```python
from build123d import *

# Parameters (mm, degrees)
SKETCH1_W                = 36
SKETCH1_H                = 120
BOSS_EXTRUDE1_DEPTH      = 1
F_4_0_4_DIAMETER_HOLE2_D = 4
F_4_0_4_DIAMETER_HOLE3_D = 4
F_4_0_4_DIAMETER_HOLE1_D = 4
BOSS_EXTRUDE2_DEPTH      = 1
FILLET1_R                = 4


with BuildPart() as part:
    # Sketch1 → Boss-Extrude1 (new body)
    with BuildSketch(Plane(origin=(0, 0, 0), x_dir=(0, 0, -1), z_dir=(1, 0, 0))):
        with Locations((0, -60)):
            Rectangle(SKETCH1_W, SKETCH1_H)
    extrude(amount=BOSS_EXTRUDE1_DEPTH)

    # Ø4.0 (4) Diameter Hole2 (through all)
    with Locations(Plane.ZY):
        with Locations((-10, -8), (10, -8)):
            Hole(F_4_0_4_DIAMETER_HOLE2_D / 2)

    # Ø4.0 (4) Diameter Hole3 (through all)
    with Locations(Plane.ZY):
        with Locations((-13, -17), (13, -17)):
            Hole(F_4_0_4_DIAMETER_HOLE3_D / 2)

    # Ø4.0 (4) Diameter Hole1 (through all)
    with Locations(Plane(origin=(1, 0, 0), x_dir=(0, 0, -1), z_dir=(1, 0, 0))):
        with Locations((6, -114), (-6, -114), (6, -104), (-6, -104), (6, -94), (-6, -94), (6, -84), (-6, -84), (6, -74), (-6, -74), (6, -64), (-6, -64), (6, -54), (-6, -54), (6, -44), (-6, -44), (6, -34), (-6, -34)):
            Hole(F_4_0_4_DIAMETER_HOLE1_D / 2)

    # Sketch9 → Boss-Extrude2 (add)
    with BuildSketch(Plane.ZY):
        with BuildLine():
            Line((18, -23.35), (23.178427125, -28.528427125))
            ThreePointArc((23.178427125, -28.528427125), (24.04551813, -29.82612052), (24.35, -31.356854249))
            Line((24.35, -31.356854249), (24.35, -116))
            ThreePointArc((24.35, -116), (23.178427125, -118.828427125), (20.35, -120))
            Line((20.35, -120), (18, -120))
            Line((18, -120), (18, -23.35))
        make_face()
        with BuildLine():
            Line((-18, -23.35), (-23.178427125, -28.528427125))
            ThreePointArc((-23.178427125, -28.528427125), (-24.04551813, -29.82612052), (-24.35, -31.356854249))
            Line((-24.35, -31.356854249), (-24.35, -116))
            ThreePointArc((-24.35, -116), (-23.178427125, -118.828427125), (-20.35, -120))
            Line((-20.35, -120), (-18, -120))
            Line((-18, -120), (-18, -23.35))
        make_face()
    extrude(amount=-BOSS_EXTRUDE2_DEPTH)

    # Fillet1
    fillet1_edges = [part.edges().sort_by_distance(p)[0] for p in [
        (0.5, 0, 18),
        (0.5, 0, -18),
    ]]
    fillet(fillet1_edges, radius=FILLET1_R)


solid = part.part
```
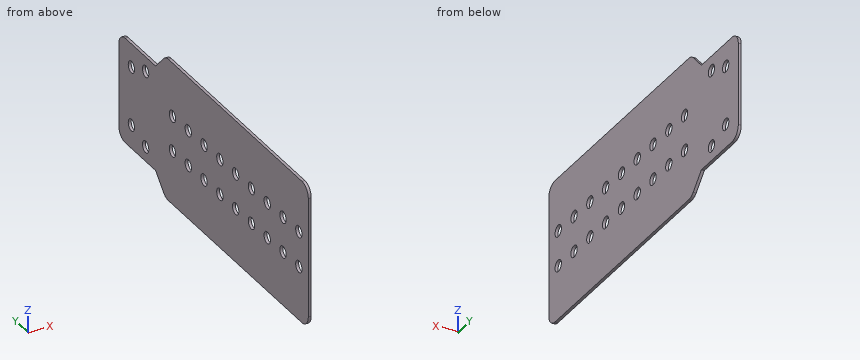
Read the model definition and answer for the solid it produces. Units are mm, in the model's axes. Give positions to 0.01 mm unless a question says otherwise; leave off trailing zeros. Write each loop counter-clockwise with the first axis right and the second up, starting at its lowest first coordinate (ties: lowest second). Pieces come first, ordered by that corner, then holes. Notation, with made-up numbers: (37.5, 58) -> (81.5, 58) arc R34 cw to (81.5, 97) -> close; hole circle Ø9 at (86.25, 7.5). An arc over 180 degrees is marked (long way). Answer as a JSON object with one key per item and string values.
1) Section A-A on y = -84 is taken. Write down the section's boundary in (x, z), then the cut area to 3 significant figures.
Findings below:
{"outline": "(0, -24.35) -> (1, -24.35) -> (1, -8) -> (0, -8) -> close; (0, -4) -> (1, -4) -> (1, 4) -> (0, 4) -> close; (0, 8) -> (1, 8) -> (1, 24.35) -> (0, 24.35) -> close", "area": "40.7 mm^2"}
2) Section C-C on y = -11.5 is taken. Write down the section's boundary in (x, z).
Findings below:
{"outline": "(0, -18) -> (1, -18) -> (1, 18) -> (0, 18) -> close"}
3) Section B-B on z = 6 is taken. Count the separate pieces of the cut face and the enclosed holes in it, then the cut area to 3 significant figures.
Findings below:
{"separate pieces": "10", "enclosed holes": "0", "area": "84.0 mm^2"}
4) Flat-ended cylindrical pins translate along their axes: pin 1 Ø8 at (y, z) = (-106, 6) entering from -X; pin 2 Ø3.5 at (y, z) = (-64, -6) entering from +X. Find the tip coordinate at first contact, or state that the pin passes through.
Findings below:
{"pin 1": "stops at x = 0", "pin 2": "passes through"}
5) Straight lines are drawn through the part: probe 1 along Z at (x, y) = (0.85, -73.5); probe 2 along Y at (x, z) = (0.45, 13); probe 3 along Y at (x, z) = (0.45, 9). For each, find the intervals that lie inside material, in ascending order. Write a range as from..to.
Findings below:
{"probe 1": "z = -24.35..-7.94, -4.06..4.06, 7.94..24.35", "probe 2": "y = -120..-19, -15..0", "probe 3": "y = -120..-9.73, -6.27..0"}
